Input: part model. Units: mm. Frame: model coordinates. A direction names the side the tool comes from. Give positions to 0.01 mm unless a question says otherwise; leave off trailing zeros. Order: outer loops, then holes, each group sorted by start corner. A loop starts at its lowest first (then second) coordinate and runs counter-clockwise, first axis right, second up. Notation, with made-up numbers: (41, -28) - (88, -28) arc R25 cw to (88, 7) - close; hole circle Ø5 at (45, 46). An arc over 180 degrees is marked (long way). Answer in a Markdown table with one row per item. Add a question column.
from build123d import *

# Parameters (mm, degrees)
SKETCH1_W           = 29
SKETCH1_H           = 5
BOSS_EXTRUDE1_DEPTH = 105
SKETCH2_R           = 7.5
CUT_EXTRUDE1_DEPTH  = 105
BOSS_EXTRUDE2_DEPTH = 5


with BuildPart() as part:
    # Sketch1 → Boss-Extrude1 (new body)
    with BuildSketch(Plane(origin=(0, 0, 0), x_dir=(0, 0, -1), z_dir=(1, 0, 0))):
        Rectangle(SKETCH1_W, SKETCH1_H)
    extrude(amount=BOSS_EXTRUDE1_DEPTH)

    # Sketch2 → Cut-Extrude1 (cut)
    with BuildSketch(Plane.XZ.offset(2.5)):
        with Locations(Location((20, 0, 0), (0, 0, 270))):
            Circle(SKETCH2_R)
        with Locations(Location((40, 0, 0), (0, 0, 270))):
            Circle(SKETCH2_R)
        with Locations(Location((60, 0, 0), (0, 0, 270))):
            Circle(SKETCH2_R)
        with Locations(Location((80, 0, 0), (0, 0, 270))):
            Circle(SKETCH2_R)
    extrude(amount=-CUT_EXTRUDE1_DEPTH, mode=Mode.SUBTRACT)

    # Sketch3 → Boss-Extrude2 (add)
    with BuildSketch(Plane.XZ.offset(2.5)):
        with BuildLine():
            Line((105, 14.5), (105, 10))
            ThreePointArc((105, 10), (115, 0), (105, -10))
            Line((105, -10), (105, -14.5))
            ThreePointArc((105, -14.5), (119.5, 0), (105, 14.5))
        make_face()
    extrude(amount=-BOSS_EXTRUDE2_DEPTH)


solid = part.part
Q1. Access query for faces 4 (the flat face through (105, 0, 0)), 5 (the flat face through (52, 0, -14.5)). Directions: +Z, -Z, +X, -X, +Y, -Y. A direction counts if a zero-diameter tool reaches every point of the face in a straight line with its end or side. Return the directions, or none.
Q2. Section D-D, the plane x = 62.5. Return loops of the section in (y, z).
Q3. Contact query for flat-ended pins moving along their axis: P1, Ø17, axis at x = 80, z = 0, coming from the -Y side; P2, Ø1.5, axis at y = -1, z = -10, coming from the +X side. Output: stop coordinate, or through.
Q4. Section A-A, the plane x = 20. Return loops of the section in (y, z), then the cut area to 3 significant figures.
Q5. Pull-direction query (X, two-part tool) for faces 1 (the flat face through (52, 0, 14.5)), 2 (the cylindrical face through (32.68, -0.04, 1.63)), 3 (the flat face through (0, 0, 0)); classes: +X half, -X half, draft (parallel to the pull), parting line (faces both ways), or undercut.
Q6. Section B-B, the plane z = 0. Return loops of the section in (x, y).
Q7. Section C-C, the plane y = 1.2. Return loops of the section in (x, z).
Q8. Line query: probe 1 along X at (y, z) = (0.35, 0); probe 2 along X at (y, z) = (-2.15, -3.5); probe 3 along Z at (x, y) = (38, 1.65). Output: solid intervals per line, ascending.
Computed:
| question | item | result |
|---|---|---|
| 1 | face 4 | +Y, -Y |
| 1 | face 5 | -Z, +X, -X, +Y, -Y |
| 2 | outline | (-2.5, -14.5) - (2.5, -14.5) - (2.5, -7.07) - (-2.5, -7.07) - close; (-2.5, 7.07) - (2.5, 7.07) - (2.5, 14.5) - (-2.5, 14.5) - close |
| 3 | P1 | stops at y = -2.5 |
| 3 | P2 | stops at x = 116.17 |
| 4 | outline | (-2.5, -14.5) - (2.5, -14.5) - (2.5, -7.5) - (-2.5, -7.5) - close; (-2.5, 7.5) - (2.5, 7.5) - (2.5, 14.5) - (-2.5, 14.5) - close |
| 4 | area | 70.0 mm^2 |
| 5 | face 1 | draft |
| 5 | face 2 | undercut |
| 5 | face 3 | -X half |
| 6 | outline | (0, -2.5) - (12.5, -2.5) - (12.5, 2.5) - (0, 2.5) - close; (27.5, -2.5) - (32.5, -2.5) - (32.5, 2.5) - (27.5, 2.5) - close; (47.5, -2.5) - (52.5, -2.5) - (52.5, 2.5) - (47.5, 2.5) - close; (67.5, -2.5) - (72.5, -2.5) - (72.5, 2.5) - (67.5, 2.5) - close; (87.5, -2.5) - (105, -2.5) - (105, 2.5) - (87.5, 2.5) - close; (115, -2.5) - (119.5, -2.5) - (119.5, 2.5) - (115, 2.5) - close |
| 7 | outline | (0, -14.5) - (105, -14.5) arc R14.5 ccw to (105, 14.5) - (0, 14.5) - close; hole circle Ø15 at (20, 0); hole circle Ø15 at (40, 0); hole circle Ø15 at (60, 0); hole circle Ø15 at (80, 0); hole (105, -10) arc R10 ccw to (105, 10) - close |
| 8 | probe 1 | x = 0 to 12.5, 27.5 to 32.5, 47.5 to 52.5, 67.5 to 72.5, 87.5 to 105, 115 to 119.5 |
| 8 | probe 2 | x = 0 to 13.37, 26.63 to 33.37, 46.63 to 53.37, 66.63 to 73.37, 86.63 to 105, 114.37 to 119.07 |
| 8 | probe 3 | z = -14.5 to -7.23, 7.23 to 14.5 |
